```python
from build123d import *

# Parameters (mm, degrees)
BOSS_EXTRUDE1_DEPTH = 5.6388


with BuildPart() as part:
    # Sketch5 → Boss-Extrude1 (new body)
    with BuildSketch(Plane.XY):
        with BuildLine():
            Line((-111.565879557, 73.61243575), (-112.004630057, 73.61243575))
            Line((-112.004630057, 73.61243575), (-112.004630057, 74.86243575))
            Line((-112.004630057, 74.86243575), (-80.192037686, 106.675))
            Line((-80.192037686, 106.675), (80.192037686, 106.675))
            Line((80.192037686, 106.675), (112.004630057, 74.86243575))
            Line((112.004630057, 74.86243575), (112.004630057, 73.61243575))
            Line((112.004630057, 73.61243575), (111.565879557, 73.61243575))
            ThreePointArc((111.565879557, 73.61243575), (108.004630057, 72.36243575), (111.565879557, 71.11243575))
            Line((111.565879557, 71.11243575), (112.004630057, 71.11243575))
            Line((112.004630057, 71.11243575), (112.004630057, -100.425))
            Line((112.004630057, -100.425), (111.565879557, -100.425))
            ThreePointArc((111.565879557, -100.425), (108.004630057, -101.675), (111.565879557, -102.925))
            Line((111.565879557, -102.925), (112.004630057, -102.925))
            Line((112.004630057, -102.925), (112.004630057, -106.675))
            Line((112.004630057, -106.675), (-112.004630057, -106.675))
            Line((-112.004630057, -106.675), (-112.004630057, -102.925))
            Line((-112.004630057, -102.925), (-111.565879557, -102.925))
            ThreePointArc((-111.565879557, -102.925), (-108.004630057, -101.675), (-111.565879557, -100.425))
            Line((-111.565879557, -100.425), (-112.004630057, -100.425))
            Line((-112.004630057, -100.425), (-112.004630057, 71.11243575))
            Line((-112.004630057, 71.11243575), (-111.565879557, 71.11243575))
            ThreePointArc((-111.565879557, 71.11243575), (-108.004630057, 72.36243575), (-111.565879557, 73.61243575))
        make_face()
    extrude(amount=BOSS_EXTRUDE1_DEPTH)


solid = part.part
```
The model under review builds one solid part; all positions refer to its coordinate system, in mm. Round coordinates to 2 decimals unless told otherwise and drop trailing zeros. Order: outer loops, then holes, each group sorted by start corner. A loop starts at its lowest first (then second) coordinate and runs counter-clockwise, first axis right, second up.
(1) For P1, Ø0.5, axis at x = 111.5, z = 2.5, coming from the +Y side; P2, Ø0.5, axis at x = 112, z = 2.5, coming from the +Y side, all flat-tipped, find the tip position at first contact; note any pin that passes through.
Working result:
P1: stops at y = 75.62
P2: stops at y = 75.12
(2) Take a section at A-A, the plane z = 3.2. State the section outline as (x, y) points (3 decimals).
Working result:
outline: (-112.005, -106.675) - (112.005, -106.675) - (112.005, -102.925) - (111.566, -102.925) arc R2 cw (long way) to (111.566, -100.425) - (112.005, -100.425) - (112.005, 71.112) - (111.566, 71.112) arc R2 cw (long way) to (111.566, 73.612) - (112.005, 73.612) - (112.005, 74.862) - (80.192, 106.675) - (-80.192, 106.675) - (-112.005, 74.862) - (-112.005, 73.612) - (-111.566, 73.612) arc R2 cw (long way) to (-111.566, 71.112) - (-112.005, 71.112) - (-112.005, -100.425) - (-111.566, -100.425) arc R2 cw (long way) to (-111.566, -102.925) - (-112.005, -102.925) - close
(3) Wall thickness on L1, parallel to Y at x = -99, z = 3.6 (3 decimals); L2, parallel to X at y = 84.5, z = 0.75; L3, parallel to X at y = 90, z = 4.85: over which ranges is each line inside the solid? List them lowest first.
Working result:
L1: y = -106.675 to 87.867
L2: x = -102.37 to 102.37
L3: x = -96.87 to 96.87
